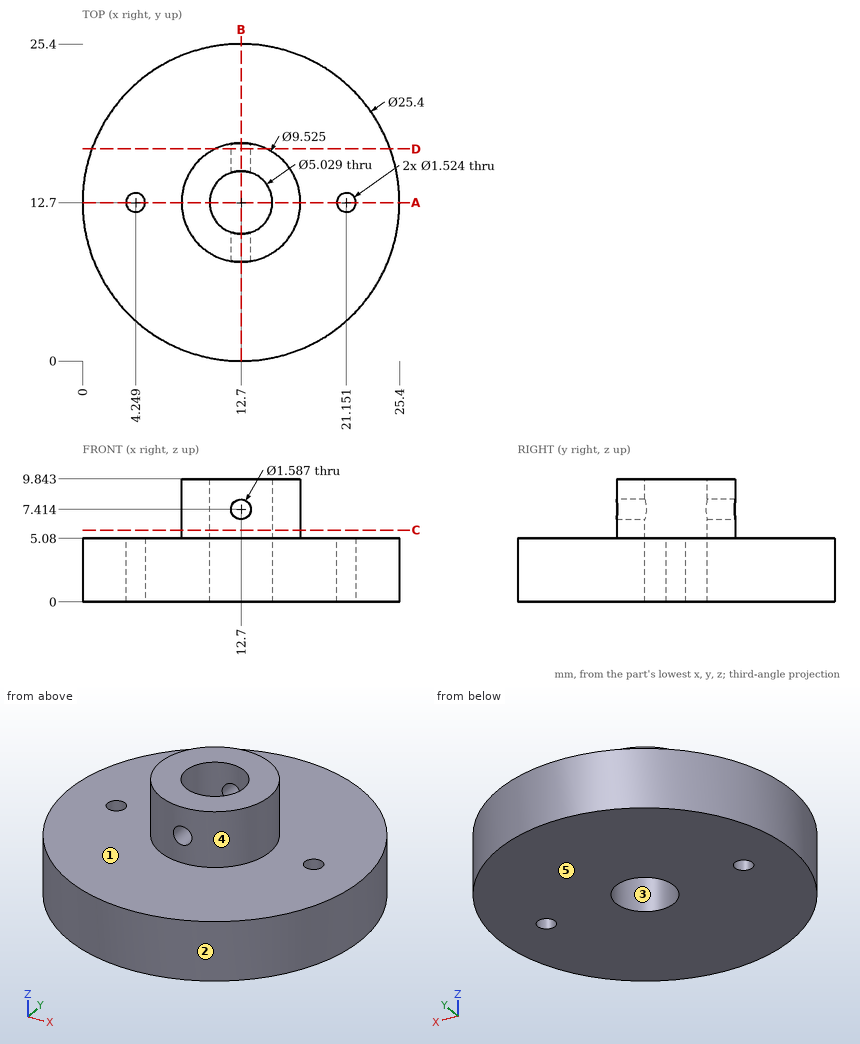
Drawing for the job (mm, zero at the part's lowest x, y, z). A direction names the side the tool comes from. Give positions to 0.01 mm unless a question says otherwise; leave off trailing zeros. Order: outer loops, then holes, each group sorted by start corner. A loop starts at its lowest first (then second) coordinate and runs counter-clockwise, first axis right, second up. Notation, with made-up numbers: M -18,-10.75 L 25,-10.75 A12 ccw 25,11.25 Z; hole C 19,77.5 d2. An arc over 180 degrees is marked long. Use a Markdown table: item, result. Add a question column.
(1) Saw through at C-C, the plane z = 5.75. Give the cut face in (x, y) (1 decimal).
(2) Drop flat-ended pins along their axis: P1, Ø1.2, axis at x = 4.25, y = 12.7, coming from the -Z side; P2, Ø1, axis at x = 15.5, z = 4, coming from the +Y side; P3, Ø2.5, axis at x = 12.7, z = 7.41, coming from the -Y side; P4, Ø5, axis at x = 21.5, z = 1.5, coming from the +Y side. Give the stop position or say it passes through.
(3) Saw through at A-A, the plane y = 12.7. Give the cut face in (x, z) (1 decimal).
(4) 3-axis set-ups, long thin cutter, end or side, ignore diameter. For the marked faces 4 and 5: which of +Z, -Z, +X, -X, +Y, -Y reach the whole face in a straight line?
(5) Saw through at D-D, the plane y = 17. Give the cut face in (x, z), and give its area (3 significant figures).
(6) Saw through at B-B, the plane x = 12.7. Give the cut face in (y, z) (1 decimal).
(7) Mould opens along X. For the marked faces 1, 2 and 3 say: +X half, -X half, draft (parallel to the pull), parting line (faces both ways), or undercut.
(8) Probe line 1 along Z through (x, y) = (12.7, 16.45); line 2 along X through (y, z) = (12.5, 4.5) (1 decimal); line 3 along Y through (x, z) = (20.5, 1.25) (1 decimal). List the from-to ranges inside material, lowest first. Write a range as [from, to].
Answer key:
| question | item | result |
|---|---|---|
| 1 | outline | C 12.7,12.7 d9.5; hole C 12.7,12.7 d5 |
| 2 | P1 | through |
| 2 | P2 | y = 25.19 |
| 2 | P3 | y = 7.94 |
| 2 | P4 | y = 23.73 |
| 3 | outline | M 0,0 L 3.5,0 L 3.5,5.1 L 0,5.1 Z; M 5,0 L 10.2,0 L 10.2,9.8 L 7.9,9.8 L 7.9,5.1 L 5,5.1 Z; M 15.2,0 L 20.4,0 L 20.4,5.1 L 17.5,5.1 L 17.5,9.8 L 15.2,9.8 Z; M 21.9,0 L 25.4,0 L 25.4,5.1 L 21.9,5.1 Z |
| 4 | face 4 | +Z |
| 4 | face 5 | -Z, +X, -X, +Y, -Y |
| 5 | outline | M 0.75,0 L 24.65,0 L 24.65,5.08 L 14.75,5.08 L 14.75,9.84 L 10.65,9.84 L 10.65,5.08 L 0.75,5.08 Z; hole C 12.7,7.41 d1.59 |
| 5 | area | 139 mm^2 |
| 6 | outline | M 0,0 L 10.2,0 L 10.2,6.6 L 7.9,6.6 L 7.9,5.1 L 0,5.1 Z; M 7.9,8.2 L 10.2,8.2 L 10.2,9.8 L 7.9,9.8 Z; M 15.2,0 L 25.4,0 L 25.4,5.1 L 17.5,5.1 L 17.5,6.6 L 15.2,6.6 Z; M 15.2,8.2 L 17.5,8.2 L 17.5,9.8 L 15.2,9.8 Z |
| 7 | face 1 | draft |
| 7 | face 2 | parting line |
| 7 | face 3 | undercut |
| 8 | line 1 | [0, 6.62], [8.21, 9.84] |
| 8 | line 2 | [0, 3.5], [5, 10.2], [15.2, 20.4], [21.9, 25.4] |
| 8 | line 3 | [2.7, 12.3], [13.1, 22.7] |
